Build history of the part. All positions in model axes, mm. Round coordinates to 2 decimals unless told otherwise and drop trailing zeros. Loops run counter-clockwise (first coordinate to the right, second up) from the corner with the lowest first, then second, coordinate; pieces in that order, holes last. Notation, with made-up numbers: (24.5, -6) - (47.5, -6) arc R29 ccw to (47.5, 18) - close; hole circle Ø4 at (-8.75, 57). An arc over 180 degrees is marked (long way). Put each result on its own line as item: value. Start each with the question number.
from build123d import *

# Parameters (mm, degrees)
BOSS_EXTRUDE1_DEPTH = 3
FILLET1_R           = 25.4
SKETCH3_R           = 28.75
CUT_EXTRUDE1_DEPTH  = 214.615601591
CIRPATTERN1_COUNT   = 4


with BuildPart() as part:
    # Sketch2 → Boss-Extrude1 (new body)
    with BuildSketch(Plane(origin=(0, 0, 0), x_dir=(1, 0, 0), z_dir=(0, 1, 0))):
        with BuildLine():
            ThreePointArc((-212.132034356, 212.132034356), (0, 126.199665585), (212.132034356, 212.132034356))
            ThreePointArc((212.132034356, 212.132034356), (126.199665585, 0), (212.132034356, -212.132034356))
            ThreePointArc((212.132034356, -212.132034356), (0, -126.199665585), (-212.132034356, -212.132034356))
            ThreePointArc((-212.132034356, -212.132034356), (-126.199665585, 0), (-212.132034356, 212.132034356))
        make_face()
    extrude(amount=BOSS_EXTRUDE1_DEPTH)

    # Fillet1
    fillet1_edges = [part.edges().sort_by_distance(p)[0] for p in [
        (212.132034356, 1.5, -212.132034356),
        (212.132034356, 1.5, 212.132034356),
        (-212.132034356, 1.5, 212.132034356),
        (-212.132034356, 1.5, -212.132034356),
    ]]
    fillet(fillet1_edges, radius=FILLET1_R)

    # Sketch3 → Cut-Extrude1 (cut, through all)
    with BuildSketch(Plane(origin=(0, 3, 0), x_dir=(1, 0, 0), z_dir=(0, 1, 0))):
        with Locations(Location((90, 0, 0), (0, 0, 270))):
            Circle(SKETCH3_R)
    cut_extrude1 = extrude(amount=-CUT_EXTRUDE1_DEPTH, mode=Mode.SUBTRACT)

    # CirPattern1: Cut-Extrude1 ×4 about axis
    cirpattern1_axis = Axis((0, 0, 0), (0, 1, 0))
    for i in range(1, CIRPATTERN1_COUNT):
        add(cut_extrude1.rotate(cirpattern1_axis, i * 360 / CIRPATTERN1_COUNT), mode=Mode.SUBTRACT)


solid = part.part
1) Slice it at B-B, the plane z = 0. Write the cut outline in (x, y), and give its area (3 significant figures).
2) Pull direction Z, two halves, no side cores. Call faces 1 (the face through (1.666, 1.479, 126.204)), 2 (the face through (126.204, 1.479, -1.666)), 3 (the face through (13.266, 1.521, -64.494)), 4 (the face through (2, 3, -2)): pulls with the +Z half, pulls with the -Z half, needs draft (parallel to the pull), parting line crosses it, or undercut.
3) Slice it at C-C, the plane z = 90. Write the cut outline in (x, y), and give its area (3 significant figures).
4) Slice it at A-A, the plane x = 0. Write the cut outline in (y, z), and give its area (3 significant figures).
5) Slice it at D-D, the plane x = 90. Write the cut outline in (y, z), and give its area (3 significant figures).
6) Drop flat-ended pins along their axis: pin 1 Ø1.5 at (x, y) = (45.5, 2) entering from +Z; pin 2 Ø6 at (x, z) = (113.5, 28) entering from -Y; pin 3 Ø1 at (x, y) = (95, 1.5) entering from -Z. Give the stop position or say it passes through.
7) Drill centre lines: line 1 (Z direction, x = 0, y = 2); line 2 (Z direction, x = -16, y = 1.4); line 3 (X direction, y = 2.5, z = 26). Where is each one in solid material? Low to high. Write a range as [from, to].
Taken from the geometry:
1. outline: (-126.2, 0) - (-118.75, 0) - (-118.75, 3) - (-126.2, 3) - close; (-61.25, 0) - (61.25, 0) - (61.25, 3) - (-61.25, 3) - close; (118.75, 0) - (126.2, 0) - (126.2, 3) - (118.75, 3) - close
1. area: 412 mm2
2. face 1: pulls with the +Z half
2. face 2: undercut
2. face 3: undercut
2. face 4: needs draft
3. outline: (-139.79, 0) - (-28.75, 0) - (-28.75, 3) - (-139.79, 3) - close; (28.75, 0) - (139.79, 0) - (139.79, 3) - (28.75, 3) - close
3. area: 666 mm2
4. outline: (0, -126.2) - (3, -126.2) - (3, -118.75) - (0, -118.75) - close; (0, -61.25) - (3, -61.25) - (3, 61.25) - (0, 61.25) - close; (0, 118.75) - (3, 118.75) - (3, 126.2) - (0, 126.2) - close
4. area: 412 mm2
5. outline: (0, -139.79) - (3, -139.79) - (3, -28.75) - (0, -28.75) - close; (0, 28.75) - (3, 28.75) - (3, 139.79) - (0, 139.79) - close
5. area: 666 mm2
6. pin 1: stops at z = 129.73
6. pin 2: stops at y = 0
6. pin 3: stops at z = -141.55
7. line 1: z = [-126.2, -118.75], [-61.25, 61.25], [118.75, 126.2]
7. line 2: z = [-126.62, -113.89], [-66.11, 66.11], [113.89, 126.62]
7. line 3: x = [-127.31, -102.27], [-77.73, 77.73], [102.27, 127.31]
